```python
from build123d import *

# Parameters (mm, degrees)
F1_DEPTH = 12.5
F2_R     = 5.5
F3_DEPTH = 25.001
F4_SIZE  = 5


with BuildPart() as f1:
    # F0 (on Top) → F1 (new body, symmetric)
    with BuildSketch(Plane.XY):
        Polygon((102.5, 15), (-125.5, 15), (-125.5, -15), (125.5, -15), (125.5, 15), (114.5, 15), (114.5, -5), (102.5, -5), align=None)
    extrude(amount=F1_DEPTH, both=True)

    # F2 (on face) → F3 (cut, through all)
    with BuildSketch(Plane.XY.offset(12.5)):
        with Locations((-103.5, 0)):
            Circle(F2_R)
    extrude(amount=-F3_DEPTH, mode=Mode.SUBTRACT)

    # F4
    f4_edges = [f1.edges().sort_by_distance(p)[0] for p in [
        (102.5, -5, 0),
        (114.5, -5, 0),
    ]]
    chamfer(f4_edges, length=F4_SIZE)


solid = f1.part
```
Verification items for the finished model (mm, model axes). A direction names the side the tool comes from. Give positions to 0.01 mm unless a question says otherwise; leave off trailing zeros. Write each loop counter-clockwise with the first axis right and the second up, starting at its lowest first coordinate (ties: lowest second). Pieces come first, ordered by that corner, then holes. Notation, with made-up numbers: (49.5, -23) - (108.5, -23) arc R27 ccw to (108.5, 10) - close; hole circle Ø8 at (63.25, 11.5). An arc over 180 degrees is marked (long way). Put each result on its own line as item: value.
Q1. Section check C-C on z = -6. Record the cut outline in (x, y), and give its area (3 significant figures).
Result:
outline: (-125.5, -15) - (125.5, -15) - (125.5, 15) - (114.5, 15) - (114.5, 0) - (109.5, -5) - (107.5, -5) - (102.5, 0) - (102.5, 15) - (-125.5, 15) - close; hole circle Ø11 at (-103.5, 0)
area: 7,220 mm2
Q2. Scan lines: probe 1 along Y at (x, z) = (-103.5, 2.75); probe 2 along X at (y, z) = (7.5, -1); probe 3 along X at (y, z) = (-1.25, 6). Record each from-to range of solid material in increasing order. Write a range as from..to.
Result:
probe 1: -15..-5.5, 5.5..15
probe 2: -125.5..102.5, 114.5..125.5
probe 3: -125.5..-108.86, -98.14..103.75, 113.25..125.5
Q3. Set-up check for faces 4 (the face through (114.5, 8, 0)), 5 (the face through (-2, 0, -12.5)): record each of +Z, -Z, +X, -X, +Y, -Y from which the full face is reachable in a straight line by a thin tool's end or side.
Result:
face 4: +Z, -Z, +Y
face 5: -Z, +X, -X, +Y, -Y
Q4. Section check B-B on x = -103.5. Record the cut outline in (y, z).
Result:
outline: (-15, -12.5) - (-5.5, -12.5) - (-5.5, 12.5) - (-15, 12.5) - close; (5.5, -12.5) - (15, -12.5) - (15, 12.5) - (5.5, 12.5) - close
Q5. Depth check by flat-ended pin: P1, Ø2, axis at x = 108, z = 0.5, coming from the +Y side. Enter the tip coordinate at first touch or a pass-through.
Result:
P1: y = -4.5
Q6. Section check A-A on y = 12. Record the cut outline in (x, z), and give its area (4 significant figures).
Result:
outline: (-125.5, -12.5) - (102.5, -12.5) - (102.5, 12.5) - (-125.5, 12.5) - close; (114.5, -12.5) - (125.5, -12.5) - (125.5, 12.5) - (114.5, 12.5) - close
area: 5,975 mm2
Q7. Mould release check, pull along Y, two halves, no side actions. Record for faces 1 (the face through (-2, -15, 0)), 2 (the face through (-109, 0, 0)), 3 (the face through (-2, 0, 12.5)): released by +Y, released by -Y, zero draft, split by the parting line, or undercut.
Result:
face 1: released by -Y
face 2: undercut
face 3: zero draft
